Design review of the part built by this model. Coordinates are the model's own, in mm. Face numbers are marked on the shaded views. A direction names the side the tool comes from. Give positions to 0.01 mm unless a question says otherwise; leave off trailing zeros. Order: outer loops, then holes, each group sorted by start corner. A loop starts at its lowest first (then second) coordinate and runs counter-clockwise, first axis right, second up. Notation, with made-up numbers: (-38, 71.5) -> (8, 71.5) arc R19 cw to (8, 83.5) -> close; hole circle Ø6 at (-17, -24.75). An arc over 180 degrees is marked (long way). One line per item, written item: value. Start each with the question number.
1) Tool access review of the marked faces 1 and 2: name each direction out of +Z, -Z, +X, -X, +Y, -Y from which nothing blocks a thin tool from reaching the whole face with its end or side.
2) The part is to be moulded in two halves that separate along Y. For the marked faces 3, 4 and 5, say which applies: released by +Y, released by -Y, zero draft, split by the parting line, or undercut.
3) Consider section A-A (y = 1). State the section outline as (x, z) points.
4) For pin 1 (1 mm diameter, centred on x = 0, y = 11, fed in from -Z), flat-tipped, find the tip position at first contact; note if it passes through.
5) Wall thickness on line 1 along X through (y, z) = (5, 0); line 2 along Y through (x, z) = (-2.25, -1.25): over which ranges is each line inside the solid? List them lowest first. Write a range as from..to.
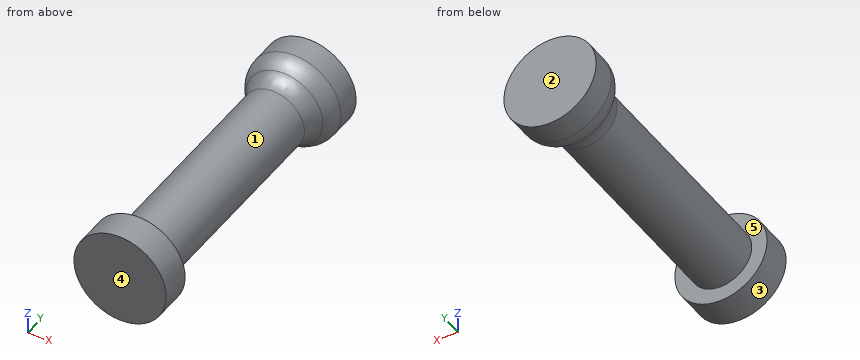
from build123d import *

# Parameters (mm, degrees)
SKETCH1_R           = 2
ROD_EXTRUSION_DEPTH = 15
SKETCH2_R           = 3
BOSS_EXTRUDE2_DEPTH = 3
FILLET3_R           = 1.5
FILLET4_R           = 1.5
INNER_START         = 2
SKETCH3_R           = 3
INNER_TIP_DEPTH     = 2


with BuildPart() as part:
    # Sketch1 → rod extrusion (new body)
    with BuildSketch(Plane(origin=(0, 0, 0), x_dir=(1, 0, 0), z_dir=(0, 1, 0))):
        with Locations(Location((0, 0, 0), (0, 0, 270))):
            Circle(SKETCH1_R)
    extrude(amount=ROD_EXTRUSION_DEPTH)

    # Sketch2 → Boss-Extrude2 (add)
    with BuildSketch(Plane(origin=(0, 15, 0), x_dir=(1, 0, 0), z_dir=(0, 1, 0))):
        with Locations(Location((0, 0, 0), (0, 0, 270))):
            Circle(SKETCH2_R)
    extrude(amount=BOSS_EXTRUDE2_DEPTH)

    # Fillet3
    # the kernel refuses this fillet: 1.5 mm, written as the material it takes off along each edge
    with BuildSketch(Plane(origin=(0, 15, 0), x_dir=(0, 0, 1), z_dir=(-1, 0, 0))) as fillet3_piece_1:
        with BuildLine():
            CenterArc((1.5, 1.414213562), FILLET3_R, 289.471220634, 70.528779366)
            Line((2, 0), (2.01, -0.028284271))
            ThreePointArc((2.01, -0.028284271), (2.5, -0.03), (3, -0.03))
            Line((3, -0.03), (3.03, 0))
            Line((3.03, 0), (3.03, 1.414213562))
            Line((3.03, 1.414213562), (3, 1.414213562))
        make_face()
    revolve(axis=Axis((0, 15, 0), (0, 1, 0)), mode=Mode.SUBTRACT)

    # Fillet4
    fillet4_edges = [part.edges().sort_by_distance(p)[0] for p in [
        (0, 15, -2),
    ]]
    fillet(fillet4_edges, radius=FILLET4_R)

    # Sketch3 → inner tip (add)
    with BuildSketch(Plane.XZ.offset(INNER_START)):
        with Locations(Location((0, 0, 0), (0, 0, 270))):
            Circle(SKETCH3_R)
    extrude(amount=-INNER_TIP_DEPTH)


solid = part.part
Checked values:
1. face 1: none
1. face 2: +Z, -Z, +X, -X, +Y
2. face 3: zero draft
2. face 4: released by -Y
2. face 5: undercut
3. outline: circle Ø4 at (0, 0)
4. pin 1: stops at z = -2
5. line 1: x = -2..2
5. line 2: y = -2..0, 15.37..18
